from build123d import *

# Parameters (mm, degrees)
ESQUISSE1_R        = 2.1
BOSS_EXTRU_1_DEPTH = 11


with BuildPart() as part:
    # Esquisse1 → Boss.-Extru.1 (new body)
    with BuildSketch(Plane.XY):
        with BuildLine():
            Line((-23.535533906, 3.535533906), (-3.535533906, 23.535533906))
            ThreePointArc((-3.535533906, 23.535533906), (3.535533906, 23.535533906), (3.535533906, 16.464466094))
            Line((3.535533906, 16.464466094), (-16.464466094, -3.535533906))
            ThreePointArc((-16.464466094, -3.535533906), (-23.535533906, -3.535533906), (-23.535533906, 3.535533906))
        make_face()
        with Locations((-20, 0)):
            Circle(ESQUISSE1_R, mode=Mode.SUBTRACT)
        with Locations((0, 20)):
            Circle(ESQUISSE1_R, mode=Mode.SUBTRACT)
        with BuildLine():
            Line((-17.424621202, 6.818019485), (-6.818019485, 17.424621202))
            ThreePointArc((-6.818019485, 17.424621202), (-2.575378798, 17.424621202), (-2.575378798, 13.181980515))
            Line((-2.575378798, 13.181980515), (-13.181980515, 2.575378798))
            ThreePointArc((-13.181980515, 2.575378798), (-17.424621202, 2.575378798), (-17.424621202, 6.818019485))
        make_face(mode=Mode.SUBTRACT)
    extrude(amount=BOSS_EXTRU_1_DEPTH)


solid = part.part
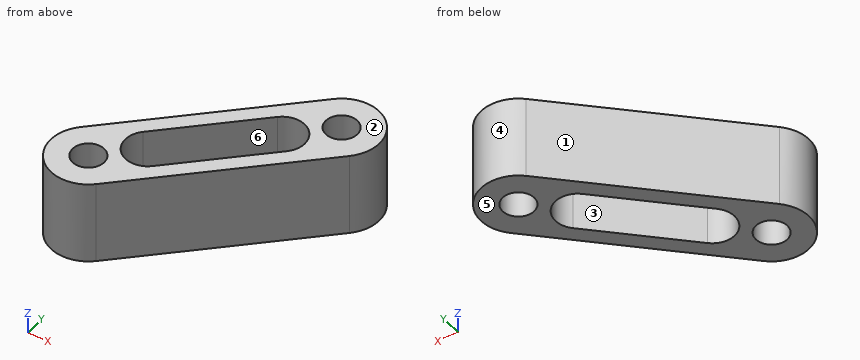
Work out the finished part from the listing and answer in its coordinate system (mm). Face numbers are marked on the shaded views. A direction names the side the tool comes from. Round coordinates to 2 decimals unless told otherwise and drop trailing zeros. Order: outer loops, then holes, each group sorted by start corner. A loop starts at its lowest first (then second) coordinate and runs counter-clockwise, first axis right, second up. Notation, with made-up numbers: M 43,31 L 84,31 A24 ccw 84,65 Z; hole C 70.5,27.5 d2. An arc over 180 degrees is marked long. Put each result on its own line as item: value. Start each with the question number.
Q1. Flat-ended cylindrical pins translate along their axes: pin 1 (2 mm diameter, centred on x = -6.5, z = 8, fed in from +Y); pin 2 (6 mm diameter, centred on x = -14.5, z = 2, fed in from -Y). Find the tip coordinate at first contact, or state that the pin passes through.
Q2. Straight lines are drawn through the part: L1, parallel to X at y = 16, z = 3.25; L2, parallel to Y at x = -14, z = 7; L3, parallel to Y at x = 0, z = 6.25. For each, find the intervals that lie inside material, in ascending order. Write a range as [from, to].
Q3. Section A-A, the plane x = -4.5 is taken. Write down the section's boundary in (y, z).
Q4. Section C-C, the plane z = 7 is taken. Write down the section's boundary in (x, y), and give its area (3 significant figures).
Q5. For a pull along X with two mould halves and no side action, classify the marked faces 1, 2, 3 and 4 as pulls with the +X half, pulls with the -X half, needs draft (parallel to the pull), parting line crosses it, or undercut.
Q6. Section B-B, the plane y = 4 is taken. Write down the section's boundary in (x, z).
Q7. A tool of negligible diameter and unlimited length cuts with its end or side. For the marked faces 5 and 6, from which of +Z, -Z, +X, -X, +Y, -Y can it reach the whole face along a straight path? Write none if from no direction.
Findings below:
1. pin 1: stops at y = 21.57
1. pin 2: stops at y = -4.33
2. L1: x = [-11.07, -8.24], [-1.78, 3.07]
2. L2: y = [-1.07, 1.99], [10.24, 13.07]
2. L3: y = [12.93, 17.9], [22.1, 25]
3. outline: M 8.43,0 L 11.26,0 L 11.26,11 L 8.43,11 Z; M 18.3,0 L 22.57,0 L 22.57,11 L 18.3,11 Z
4. outline: M -23.54,3.54 A5 ccw -16.46,-3.54 L 3.54,16.46 A5 ccw -3.54,23.54 Z; hole C -20,0 d4.2; hole M -17.42,6.82 A3 ccw -13.18,2.58 L -2.58,13.18 A3 ccw -6.82,17.42 Z; hole C 0,20 d4.2
4. area: 215 mm^2
5. face 1: pulls with the -X half
5. face 2: needs draft
5. face 3: undercut
5. face 4: parting line crosses it
6. outline: M -23.07,0 L -18.22,0 L -18.22,11 L -23.07,11 Z; M -11.76,0 L -8.93,0 L -8.93,11 L -11.76,11 Z
7. face 5: -Z, +X, -X, +Y, -Y
7. face 6: +Z, -Z
